The listing builds one solid part. Answer for the finished solid, in the listing's coordinates (mm). A direction names the side the tool comes from. Coordinates: 2 decimals unless noted, no trailing zeros. Order: outer loops, then holes, each group sorted by start corner. A loop starts at its lowest first (then second) coordinate and runs counter-clockwise, first axis right, second up. Notation, with made-up numbers: (52, 50) - (62, 50) arc R22 cw to (62, 85) - close; hole circle Ø11 at (13, 84). An arc over 180 degrees is marked (long way). Use a Markdown table: item, result. Add a question column.
Item 1: Flat-ended cylindrical pins translate along their axes: P1, Ø3.5, axis at y = 0.12, z = 52.5, coming from the -X side; P2, Ø3, axis at x = 12.5, y = -13, coming from the +Z side; P3, Ø1, axis at x = 3, z = 30.5, coming from the +Y side. Find the tip coordinate at first contact, or state that the pin passes through.
Item 2: Find the intervals of material crossed by line 1 along Y through (x, z) = (-1.15, 43.5); line 2 along Z through (x, y) = (0.5, -0.5); line 3 along Y through (x, z) = (0, 43), in increasing order.
Item 3: The part is cut by section D-D, the plane x = 5.5. Give the vertices of the cut face in (y, z), then the cut area to 3 significant figures.
Item 4: The part is cut by section B-B, the plane z = 52.5. Give the vertices of the cut face in (x, y).
Item 5: The mould has two halves that part along Y. Classify faces 3 (the cylindrical face through (2.747, 0.121, 28.028)), 4 (the flat face through (2, 0, 57)), 5 (the cylindrical face through (1.761, -1.345, 52.175)): released by +Y, released by -Y, zero draft, split by the parting line, or undercut.
Item 6: For faces 1 (the flat face through (0.8, -1, 51)), 2 (the cylindrical face through (-0.038, -0.794, 42.31)), determine the directions among +Z, -Z, +X, -X, +Y, -Y from which every point of the face is accessible in a straight line to the end or side of a thin tool.
Item 7: The part is cut by section C-C, the plane z = 27.5. Give the vertices of the cut face in (x, y), then the cut area to 3 significant figures.
Item 8: The part is cut by section A-A, the plane x = 0. Give the vertices of the cut face in (y, z).
Autodesk Inventor part; units mm, degrees
ref_plane "Work Plane1" through (0, 0, 0) normal (1, 0, 0) x (0, 1, 0)
ref_plane "XZ Plane" through (0, 0, 0) normal (0, 1, 0) x (-1, 0, 0)
ref_plane "XY Plane" through (0, 0, 0) normal (0, 0, 1) x (1, 0, 0)
sketch "Sketch1" plane through (0, 0, 0) normal (0, 1, 0) x (-1, 0, 0)
  line L0 (0, 0) -> (3, 0)
  line L1 (3, 0) -> (3, 50)
  line L2 (3, 50) -> (0, 50)
  line L3 (0, 50) -> (0, 0)
  dimension "d0" = 3
  dimension "d1" = 50
revolve "Revolution1" add sketch "Sketch1" angle 360 about axis through (0, 0, 50) along (0, 0, -1)
sketch "Sketch2" plane through (0, 0, 0) normal (0, 0, -1) x (-1, 0, 0)
  line L0 (-17.5, 17.5) -> (17.5, 17.5)
  line L1 (17.5, 17.5) -> (17.5, -17.5)
  line L2 (17.5, -17.5) -> (-17.5, -17.5)
  line L3 (-17.5, -17.5) -> (-17.5, 17.5)
  line L4 (-17.5, 17.5) -> (17.5, -17.5) construction
  line L5 (17.5, 17.5) -> (-17.5, -17.5) construction
  point P0 (0, 0)
  dimension "d6" = 35
  dimension "d7" = 35
extrude "Extrusion1" add sketch "Sketch2" against normal blind 14
sketch "Sketch3" plane through (-17.5, 17.5, 0) normal (0, 1, 0) x (1, 0, 0)
  line L0 (35, 0) -> (35, -14)
  line L1 (0, 0) -> (35, 0)
  arc A0 (0, 0) -> (35, 0) centre (17.5, 9.6825) ccw
  point P0 (17.5, 0)
  dimension "d10" = 20
  dimension "d11" = 17.5
extrude "Extrusion2" cut sketch "Sketch3" against normal through all keep common part
sketch "Sketch4" plane through (17.5, -17.5, 0) normal (1, 0, 0) x (0, 0, -1)
  line L0 (0, 35) -> (0, 0)
  line L1 (0, 35) -> (0, 0)
  arc A0 (0, 35) -> (0, 0) centre (9.6825, 17.5) ccw
  point P0 (0, 17.5)
  dimension "d14" = 20
extrude "Extrusion3" cut sketch "Sketch4" against normal through all keep common part
sketch "Sketch5" plane through (17.5, 17.5, 0) normal (0, 0, -1) x (-1, 0, 0)
  line L0 (35, 0) -> (17.5, -17.5)
  circle A0 centre (17.5, -17.5) radius 2.75
  dimension "d17" = 5.5
extrude "Extrusion4" add sketch "Sketch5" against normal blind 48
ref_plane "Work Plane1" through (0, 0, 0) normal (1, 0, 0) x (0, 1, 0)
sketch "Sketch6" plane through (0, 0, 48) normal (0, 0, 1) x (1, 0, 0)
  circle A0 centre (0, 0) radius 2.75
  line L0 (0.8, -2.6311) -> (0.8, 2.6311)
  arc A1 (0.8, -2.6311) -> (0.8, 2.6311) centre (0, 0) ccw
  point P0 (0, 0)
  dimension "d28" = 0.8
extrude "Extrusion5" add sketch "Sketch6" along normal blind 9 contours A0 L0 picked at (0.979, 0.801)
sketch "Sketch7" plane through (0.8, -2.6311, 48) normal (-1, 0, 0) x (0, 0, 1)
  circle A0 centre (4.5, 2.75) radius 1.5
  line L0 (9, 5.2621) -> (9, 0)
  circle A1 centre (-4.5, 2.75) radius 1.5
  point P0 (-48, 2.6311)
  dimension "d23" = 3
  dimension "d24" = 4.5
  dimension "d31" = 3
  dimension "d32" = 9
extrude "Extrusion6" cut sketch "Sketch7" along normal through all both and the other way through all
equation "\"d7\" = d6"
properties part number "thumper-bumper-plunger"
Solution:
| question | item | result |
|---|---|---|
| 1 | P1 | stops at x = 0.8 |
| 1 | P2 | stops at z = 6.52 |
| 1 | P3 | stops at y = 1.15 |
| 2 | line 1 | y = -2.5 to -1.38, 1.62 to 2.5 |
| 2 | line 2 | z = 0 to 42.13, 44.87 to 48 |
| 2 | line 3 | y = -2.75 to -1.3, 1.53 to 2.75 |
| 3 | outline | (-17.5, 0) - (17.5, 0) arc R20 ccw to (5.5, 9.55) - (-5.5, 9.55) arc R20 ccw to start |
| 3 | area | 251 mm2 |
| 4 | outline | (0.8, -2.63) arc R2.75 ccw to (2.38, -1.38) - (0.8, -1.38) - close; (0.8, 1.62) - (2.22, 1.62) arc R2.75 ccw to (0.8, 2.63) - close |
| 5 | face 3 | split by the parting line |
| 5 | face 4 | zero draft |
| 5 | face 5 | undercut |
| 6 | face 1 | +Z, -X, +Y, -Y |
| 6 | face 2 | +X, -X |
| 7 | outline | circle Ø5.5 at (0, 0) |
| 7 | area | 23.8 mm2 |
| 8 | outline | (-17.5, 0) - (17.5, 0) arc R20 ccw to (2.75, 10.13) - (2.75, 48) - (-2.75, 48) - (-2.75, 10.13) arc R20 ccw to start; hole circle Ø3 at (0.12, 43.5) |
